```python
from build123d import *

# Parameters (mm, degrees)
SKETCH1_W           = 71.12
SKETCH1_H           = 71.12
BOSS_EXTRUDE1_DEPTH = 50.8
SKETCH2_W           = 96.52
SKETCH2_H           = 96.52
BOSS_EXTRUDE2_DEPTH = 5.08
SKETCH3_W           = 64.77
SKETCH3_H           = 64.77
CUT_EXTRUDE1_DEPTH  = 45.72
SKETCH4_R           = 3.81
CUT_EXTRUDE2_DEPTH  = 86.08052186


with BuildPart() as part:
    # Sketch1 → Boss-Extrude1 (new body)
    with BuildSketch(Plane(origin=(0, 0, 0), x_dir=(1, 0, 0), z_dir=(0, 1, 0))):
        Rectangle(SKETCH1_W, SKETCH1_H)
    extrude(amount=BOSS_EXTRUDE1_DEPTH)

    # Sketch2 → Boss-Extrude2 (add)
    with BuildSketch(Plane(origin=(0, 0, 0), x_dir=(1, 0, 0), z_dir=(0, 1, 0))):
        Rectangle(SKETCH2_W, SKETCH2_H)
    extrude(amount=BOSS_EXTRUDE2_DEPTH)

    # Sketch3 → Cut-Extrude1 (cut)
    with BuildSketch(Plane.XZ):
        Rectangle(SKETCH3_W, SKETCH3_H)
    extrude(amount=-CUT_EXTRUDE1_DEPTH, mode=Mode.SUBTRACT)

    # Sketch4 → Cut-Extrude2 (cut, through all)
    with BuildSketch(Plane(origin=(0, 50.8, 0), x_dir=(1, 0, 0), z_dir=(0, 1, 0))):
        with Locations(Location((0, 0, 0), (0, 0, 270))):
            Circle(SKETCH4_R)
    extrude(amount=-CUT_EXTRUDE2_DEPTH, mode=Mode.SUBTRACT)


solid = part.part
```
Build history of the part. All positions in model axes, mm. A direction names the side the tool comes from. Give positions to 0.01 mm unless a question says otherwise; leave off trailing zeros. Loops run counter-clockwise (first coordinate to the right, second up) from the corner with the lowest first, then second, coordinate; pieces in that order, holes last. Notation, with made-up numbers: (-33.75, 47.5) - (16.25, 47.5) arc R20 cw to (16.25, 71.5) - close; hole circle Ø1 at (7, 17). An arc over 180 degrees is marked (long way). Use a Markdown table: item, result.
(1) Band-saw the part on B-B (z = 0). Give the cut face in (x, y) (3 decimals).
Taken from the geometry:
| item | result |
|---|---|
| outline | (-48.26, 0) - (-32.385, 0) - (-32.385, 45.72) - (-3.81, 45.72) - (-3.81, 50.8) - (-35.56, 50.8) - (-35.56, 5.08) - (-48.26, 5.08) - close; (3.81, 45.72) - (32.385, 45.72) - (32.385, 0) - (48.26, 0) - (48.26, 5.08) - (35.56, 5.08) - (35.56, 50.8) - (3.81, 50.8) - close |
(2) Pull direction Z, two halves, no side cores. Call faces 1 (the face through (-1, 3, 48.26)), 2 (the face through (-32.385, 23, 0)), 3 (the face through (35.56, 28, 0)): +Z half, -Z half, draft (parallel to the pull), parting line (faces both ways), or undercut.
Taken from the geometry:
| item | result |
|---|---|
| face 1 | +Z half |
| face 2 | undercut |
| face 3 | draft |
(3) Wall check: line 1 along X through (y, z) = (46.9, 0); line 2 along X through (y, z) = (20, 10.5) (3 decimals). Give the ranges that are in metal, low to high.
Taken from the geometry:
| item | result |
|---|---|
| line 1 | -35.56 to -3.81, 3.81 to 35.56 |
| line 2 | -35.56 to -32.385, 32.385 to 35.56 |
(4) Band-saw the part on A-A (x = 0). Give the cut face in (y, z) (3 decimals), and give its area (3 significant figures).
Taken from the geometry:
| item | result |
|---|---|
| outline | (0, -48.26) - (5.08, -48.26) - (5.08, -35.56) - (50.8, -35.56) - (50.8, -3.81) - (45.72, -3.81) - (45.72, -32.385) - (0, -32.385) - close; (0, 32.385) - (45.72, 32.385) - (45.72, 3.81) - (50.8, 3.81) - (50.8, 35.56) - (5.08, 35.56) - (5.08, 48.26) - (0, 48.26) - close |
| area | 742 mm2 |
(5) Band-saw the part on D-D (x = 11). Give the cut face in (y, z) (3 decimals).
Taken from the geometry:
| item | result |
|---|---|
| outline | (0, -48.26) - (5.08, -48.26) - (5.08, -35.56) - (50.8, -35.56) - (50.8, 35.56) - (5.08, 35.56) - (5.08, 48.26) - (0, 48.26) - (0, 32.385) - (45.72, 32.385) - (45.72, -32.385) - (0, -32.385) - close |
(6) Which spindle directions (+Z, -Z, +X, -X, +Y, -Y) get a long thin tool onto all of the face, cutting with end or side? Do faces 4 (the face through (0, 23, 32.385)), 5 (the face through (-35.56, 28, 0)), 6 (the face through (0, 28, 35.56)). Say none if no direction does.
Taken from the geometry:
| item | result |
|---|---|
| face 4 | -Y |
| face 5 | +Z, -Z, -X, +Y |
| face 6 | +Z, +X, -X, +Y |
(7) Band-saw the part on C-C (y = 31.5). Give the cut face in (x, z) (3 decimals).
Taken from the geometry:
| item | result |
|---|---|
| outline | (-35.56, -35.56) - (35.56, -35.56) - (35.56, 35.56) - (-35.56, 35.56) - close; hole (-32.385, -32.385) - (32.385, -32.385) - (32.385, 32.385) - (-32.385, 32.385) - close |
(8) Drop flat-ended pins along their axis: pin 1 Ø23 at (y, z) = (34, -8.5) entering from +X; pin 2 Ø6 at (y, z) = (36, 11) entering from -X; pin 3 Ø23 at (x, y) = (2.5, 22) entering from +Z. Give the stop position or say it passes through.
Taken from the geometry:
| item | result |
|---|---|
| pin 1 | x = 35.56 |
| pin 2 | x = -35.56 |
| pin 3 | z = 35.56 |
